```python
from build123d import *

# Parameters (mm, degrees)
ESQUISSE1_R = 0.5


with BuildPart() as part:
    # Balayage1: sweep along a curve in space
    with BuildLine() as balayage1_path:
        Line((0, 0, 0), (0, 0, 3.5))
        Line((0, 0, 3.5), (0, 44.06, 3.5))
        Line((0, 44.06, 3.5), (0, 44.06, -22.79))
        Line((0, 44.06, -22.79), (2.28, 44.06, -22.79))
        Line((2.28, 44.06, -22.79), (2.28, 44.06, -26.29))
    # Esquisse1 → Balayage1 (sweep)
    with BuildSketch(Plane(origin=(0, 0, 0), x_dir=(0, 1, 0), z_dir=(0, 0, 1))):
        Circle(ESQUISSE1_R)
    sweep(path=balayage1_path.line, transition=Transition.RIGHT)


solid = part.part
```
Model file for the job. Use its own axes, mm. A direction names the side the tool comes from. Give positions to 0.01 mm unless a question says otherwise; leave off trailing zeros. Loops run counter-clockwise (first coordinate to the right, second up) from the corner with the lowest first, then second, coordinate; pieces in that order, holes last. Notation, with made-up numbers: (70.25, 45.5) -> (123.25, 45.5) arc R27 cw to (123.25, 65.5) -> close; hole circle Ø3 at (33.5, -8.5). An arc over 180 degrees is marked (long way). Use CSV: the item, a comma, the result in double quotes. Start each with the question number.
1) Wall check: line 1 (Z direction, x = 0.1, y = 17); line 2 (Y direction, x = -0.2, z = -14.5); line 3 (Z direction, x = 0.4, y = 7.5). Give the ranges that are in metal, low to high.
2) Flat gauge pin, fed straight in: pin 1 Ø0.5 at (x, y) = (0, 0) entering from -Z. Where does the tip first touch, or does it go through?
3) Tool access for faces 1 (the flat face through (0, 0, 0)), 2 (the flat face through (2, 44, -26.29)), 3 (the cylindrical face through (-0.02, 44.56, -9.84)), 4 (the cylindrical face through (0, -0.5, 1.6)): list every direction of +Z, -Z, +X, -X, +Y, -Y with a clear straight run to the whole face (end or side of a thin tool).
4) Slice it at C-C on z = 2.5. Give the cut face in (x, y).
5) Slice it at A-A on y = 44.06. Give the cut face in (x, z), plus the area to 3 significant figures.
6) Slice it at D-D on z = -22.79. Give the cut face in (x, y).
7) Mould opens along X. For faces 5 (the cylindrical face through (0, 22, 4)), 6 (the cylindrical face through (1.16, 44.56, -22.81)) say: released by +X, released by -X, zero draft, split by the parting line, or undercut.
8) Slice it at B-B on x = 0. Give the cut face in (y, z).
Computed values:
1,line 1,"z = 3.01 to 3.99"
1,line 2,"y = 43.6 to 44.52"
1,line 3,"z = 3.2 to 3.8"
2,pin 1,"stops at z = 0"
3,face 1,"-Z, +X, -X, -Y"
3,face 2,"-Z, +X, -X, +Y, -Y"
3,face 3,"none"
3,face 4,"-Z"
4,outline,"circle Ø1 at (0, 0); circle Ø1 at (0, 44.06)"
5,outline,"(-0.5, -23.29) -> (1.78, -23.29) -> (1.78, -26.29) -> (2.78, -26.29) -> (2.78, -22.29) -> (0.5, -22.29) -> (0.5, 3.5) arc R0.5 ccw to (-0.5, 3.5) -> close"
5,area,"32.5 mm^2"
6,outline,"(0, 43.56) -> (2.28, 43.56) arc R0.5 ccw to (2.28, 44.56) -> (0, 44.56) arc R0.5 ccw to start"
7,face 5,"split by the parting line"
7,face 6,"zero draft"
8,outline,"(-0.5, 0) -> (0.5, 0) -> (0.5, 3) -> (43.56, 3) -> (43.56, -22.79) arc R0.5 ccw to (44.56, -22.79) -> (44.56, 4) -> (-0.5, 4) -> close"
